Part model, mm, in its own coordinate system. A direction names the side the tool comes from. Coordinates: 2 decimals unless noted, no trailing zeros. Loops run counter-clockwise (first coordinate to the right, second up) from the corner with the lowest first, then second, coordinate; pieces in that order, holes last. Notation, with made-up numbers: M 82,-40 L 135,-40 A20 ccw 135,-31 Z; hole C -12.75,-23.75 d10. An arc over 180 degrees is marked long. Answer as a JSON object with one key per item and string values. Group by question number.
1. 3-axis set-ups, long thin cutter, end or side, ignore diameter. For faces 1 (the face through (-34, -8, -1)), 2 (the face through (35.99, -7.49, -0.76)): which of +Z, -Z, +X, -X, +Y, -Y reach the whole face in a straight line?
2. Saw through at B-B on z = 35. Write the cut outline in (x, y).
3. Saw through at C-C on y = -8.7. Write the cut outline in (x, z).
4. Mould opens along Z. For faces 3 (the face through (-0.1, -8, -4.4)), 4 (the face through (8, -10, -8)), 5 (the face through (-8.67, -8.48, 39.05)) say: released by +Z, released by -Z, zero draft, split by the parting line, or undercut.
5. Drill centre lines: L1, parallel to Z at x = 0.5, y = -9.45; L2, parallel to Z at x = -36, y = -7.9; L3, parallel to X at y = -9.5, z = 5. Where is each one in solid material? Low to high.
6. Saw through at D-D on x = 0. Count the separate pieces of the cut face and the enclosed holes in it, then the cut area to 4 significant figures.
7. Saw through at A-A on x = -35. Write the cut outline in (y, z), then the cut area to 3 significant figures.
8. Drop flat-ended pins along their axis: pin 1 Ø3 at (x, z) = (-6.01, 6.01) entering from -Y; pin 2 Ø1.5 at (y, z) = (-8.5, 2.5) entering from -X; pin 3 Ø1.5 at (x, y) = (-22.5, -9) entering from +Z. Give the stop position or say it passes through.
Autodesk Inventor part; units mm, degrees
ref_plane "YZ Plane" through (0, 0, 0) normal (1, 0, 0) x (0, 1, 0)
ref_plane "XZ Plane" through (0, 0, 0) normal (0, 1, 0) x (-1, 0, 0)
ref_plane "XY Plane" through (0, 0, 0) normal (0, 0, 1) x (1, 0, 0)
sketch "Sketch1" plane through (0, 0, 0) normal (0, 1, 0) x (-1, 0, 0)
  circle A0 centre (0, 0) radius 30
  circle A1 centre (0, 0) radius 45
  circle A2 centre (0, 0) radius 20
  dimension "d0" = 60
  dimension "d1" = 90
  dimension "d2" = 40
extrude "Extrusion1" add sketch "Sketch1" along normal blind 20 draft -4 contours A0
sketch "Sketch2" plane through (0, 20, 0) normal (0, 1, 0) x (1, 0, 0)
  circle A0 centre (0, 0) radius 28.6015
  circle A1 centre (0, 0) radius 21.3985
extrude "Extrusion2" add sketch "Sketch2" along normal blind 20 draft 4
sketch "Sketch3" plane through (0, 40, 0) normal (0, 1, 0) x (1, 0, 0)
  circle A0 centre (0, 0) radius 40
  dimension "d7" = 80
extrude "Extrusion3" add sketch "Sketch3" along normal blind 10
sketch "Sketch4" plane through (0, 0, 0) normal (0, -1, 0) x (1, 0, 0)
  circle A0 centre (0, 0) radius 40
  dimension "d10" = 80
extrude "Extrusion4" add sketch "Sketch4" along normal blind 10
sketch "Sketch5" plane through (0, -10, 0) normal (0, -1, 0) x (1, 0, 0)
  circle A0 centre (0, 0) radius 2.25
  circle A1 centre (0, 0) radius 4.25
  circle A2 centre (0, 0) radius 10.25
  dimension "d13" = 4.5
  dimension "d16" = 8.5
  dimension "d17" = 20.5
extrude "Extrusion9" cut sketch "Sketch5" against normal blind 2 contours A2
extrude "Extrusion10" cut sketch "Sketch5" against normal blind 4 contours A0 | A1
sketch "Sketch6" plane through (0, -8, 0) normal (0, -1, 0) x (1, 0, 0)
  circle A0 centre (0, 8.5) radius 1.25
  circle A1 centre (0, 0) radius 8.5
  circle A2 centre (-6.0104, 6.0104) radius 1.25
  circle A3 centre (-8.5, 0) radius 1.25
  circle A4 centre (-6.0104, -6.0104) radius 1.25
  circle A5 centre (0, -8.5) radius 1.25
  circle A6 centre (6.0104, -6.0104) radius 1.25
  circle A7 centre (8.5, 0) radius 1.25
  circle A8 centre (6.0104, 6.0104) radius 1.25
  circle A9 centre (0, 0) radius 10.25
  line L0 (0, 8.5) -> (0, 7.25) construction
  line L1 (0, -8.5) -> (0, -7.25) construction
  line L2 (0, 7.25) -> (0, 0) construction
  point P0 (5.0639, 6.8269)
  point P1 (6.8269, 5.0639)
  dimension "d34" = 2.5
  dimension "d30" = 360
  dimension "d36" = 14.5
  dimension "d37" = 1.25
extrude "Extrusion11" cut sketch "Sketch6" against normal through all contours A0 A1 | A1 A0 | A2 A1 | A1 A2 | A8 A1 | A1 A8 | A3 A1 | A1 A3 | A7 A1 | A1 A7 | A4 A1 | A1 A4 | A6 A1 | A1 A6 | A5 A1 | A1 A5
sketch "Sketch7" plane through (0, -10, 0) normal (0, -1, 0) x (1, 0, 0)
  point P0 (0, 0)
sketch "Sketch8" plane through (0, 50, 0) normal (0, 1, 0) x (1, 0, 0)
  circle A0 centre (0, 0) radius 69.6174
extrude "Extrusion12" cut sketch "Sketch8" against normal blind 57
sketch "Sketch12" plane through (0, -10, 0) normal (0, -1, 0) x (1, 0, 0)
  circle A0 centre (0, 0) radius 4.25
  circle A1 centre (0, 0) radius 35 construction
  point P0 (0, 35)
  dimension "d57" = 70
hole "Hole2" at (0, -10, 35) direction (0, 1, 0) diameter 2.5 depth 8 tip angle 118 counterbore diameter 5 counterbore depth 2
pattern_circular "Circular Pattern2" count 4 over 360 about axis through (0, 0, 0) along (0, -1, 0) of "Hole2"
sketch "Sketch9" plane through (0, -10, 0) normal (0, -1, 0) x (1, 0, 0)
  circle A0 centre (0, 0) radius 16.7725
  circle A1 centre (0, 0) radius 4.25
  circle A2 centre (0, 0) radius 45.7596
properties part number "spool_test" material "ABS Plastic"
Outcome:
{
 "1": {"face 1": "-Y", "face 2": "+Y, -Y"},
 "2": {"outline": "M -19.36,-10 L -2.5,-10 L -2.5,-8 L -1.25,-8 L -1.25,-7 L -19.36,-7 Z; M 1.25,-8 L 2.5,-8 L 2.5,-10 L 19.36,-10 L 19.36,-7 L 1.25,-7 Z"},
 "3": {"outline": "C 0,0 d80; hole C -35,0 d5; hole C 0,0 d20.5; hole C 0,-35 d5; hole C 0,35 d5; hole C 35,0 d5"},
 "4": {"face 3": "undercut", "face 4": "zero draft", "face 5": "split by the parting line"},
 "5": {"L1": "z = -40 to -37.45, -32.55 to -10.24, 10.24 to 32.55, 37.45 to 40", "L2": "z = -17.44 to -0.75, 0.75 to 17.44", "L3": "x = -39.69 to -8.95, 8.95 to 39.69"},
 "6": {"separate pieces": "6", "enclosed holes": "0", "area": "160.5 mm²"},
 "7": {"outline": "M -10,-19.36 L -7,-19.36 L -7,-1.25 L -8,-1.25 L -8,-2.5 L -10,-2.5 Z; M -10,2.5 L -8,2.5 L -8,1.25 L -7,1.25 L -7,19.36 L -10,19.36 Z", "area": "104 mm²"},
 "8": {"pin 1": "stops at y = -8", "pin 2": "stops at x = -39.96", "pin 3": "stops at z = 33.57"}
}
